Part model, mm, in its own coordinate system. A direction names the side the tool comes from. Give positions to 0.01 mm unless a question says otherwise; leave off trailing zeros. Order: outer loops, then holes, each group sorted by start corner. A loop starts at its lowest first (then second) coordinate and runs counter-clockwise, first axis right, second up.
1. Drop flat-ended pins along their axis: pin 1 Ø4.5 at (x, z) = (4.5, -9) entering from +Y; pin 2 Ø1.5 at (x, z) = (5, 3) entering from -Y; pin 3 Ø4 at (x, y) = (6.5, 3) entering from +Z. Give the stop position or say it passes through.
2. Which spindle directions (+Z, -Z, +X, -X, +Y, -Y) get a long thin tool onto all of the face, cutting with end or side? Do faces 5 (the flat face through (4, 2, -8)), 6 (the cylindrical face through (6.54, -3.81, -10.74)), 7 (the cylindrical face through (3.642, 3.807, -12.414)). Say none if no direction does.
3. Slice it at C-C on x = 5. List the corners of the cut face in (y, z), and give its area (3 significant figures).
4. Slice it at B-B on x = 4. List the corners of the cut face in (y, z), and give its area (3 significant figures).
5. Slice it at D-D on y = 0. List the corners of the cut face in (x, z), and give its area (3 significant figures).
6. Probe line 1 (Z direction, x = 4, y = 2.75); line 2 (Z direction, x = 4, y = 3.9); line 3 (Y direction, x = 3.5, z = -12.5). List the from-to ranges inside material, lowest first.
7. Mould opens along X. For faces 1 (the flat face through (1, 4.3, -11)), 2 (the flat face through (0, -4, -5)), 3 (the cylindrical face through (5.386, -2.659, -10.262)), 4 (the flat face through (5.2, 3.3, -8.5)) say: +X half, -X half, draft (parallel to the pull), parting line (faces both ways), or undercut.
8. Slice it at A-A on z = 0. List the corners of the cut face in (x, y), and give its area (3 significant figures).
Autodesk Inventor part; units mm, degrees
ref_plane "YZ Plane" through (0, 0, 0) normal (1, 0, 0) x (0, 1, 0)
ref_plane "XZ Plane" through (0, 0, 0) normal (0, 1, 0) x (-1, 0, 0)
ref_plane "XY Plane" through (0, 0, 0) normal (0, 0, 1) x (1, 0, 0)
sketch "Sketch2" plane through (0, 0, 0) normal (1, 0, 0) x (0, 1, 0)
  arc A0 (2, -4.8) -> (-2, -4.8) centre (0, 0) ccw
  arc A1 (2, -7.4357) -> (-2, -7.4357) centre (0, 0) ccw
  line L0 (0, 0) -> (2, -4.8)
  line L1 (2, -4.8) -> (2, -7.4357)
  line L2 (2, -7.4357) -> (2, -13.4357)
  line L3 (2, -13.4357) -> (4.3, -13.4357)
  line L4 (4.3, -13.4357) -> (4.3, -6.3875)
  line L5 (0, 0) -> (0, -16.8496) construction
  line L6 (0, 0) -> (-2, -4.8)
  line L7 (-2, -4.8) -> (-2, -7.4357)
  line L8 (-2, -7.4357) -> (-2, -13.4357)
  line L9 (-2, -13.4357) -> (-4.3, -13.4357)
  line L10 (-4.3, -13.4357) -> (-4.3, -6.3875)
  line L11 (-4.3, -6.3875) -> (-2, -6.3875)
  arc A2 (0, -5.2) -> (2, -4.8) centre (0, 0) ccw
  arc A3 (0, -7.7) -> (2, -7.4357) centre (0, 0) ccw
  arc A4 (-2, -7.4357) -> (0, -7.7) centre (0, 0) ccw
  arc A5 (-2, -4.8) -> (0, -5.2) centre (0, 0) ccw
  dimension "d6" = 10.4
  dimension "d7" = 2.5
  dimension "d9" = 2
  dimension "d10" = 6
  dimension "d11" = 2.3
  dimension "d12" = 90
extrude "Extrusion1" add sketch "Sketch2" along normal blind 8 contours A0 L7 L11 A1 L1 | A1 L4 L3 L2 | L7 A1 L11 | L8 L9 L10 A1
sketch "Sketch3" plane through (0, 4.3, -6.3875) normal (0, 1, 0) x (1, 0, 0)
  line L0 (0, 7.0482) -> (0, 0)
  line L1 (0, 0) -> (8, 0)
  line L2 (8, 7.0482) -> (8, 0)
  line L3 (0, 7.0482) -> (8, 7.0482)
  circle A0 centre (4, 3.3) radius 1.5
  point P0 (0, -6.3875)
  dimension "d15" = 3
  dimension "d21" = 3.3
extrude "Extrusion2" cut sketch "Sketch3" against normal up to next contours A0
sketch "Sketch4" plane through (0, 4.3, -6.3875) normal (0, 1, 0) x (1, 0, 0)
  line L0 (0, 7.0482) -> (0, -1.5875)
  line L1 (0, -1.5875) -> (8, -1.5875)
  line L2 (8, 7.0482) -> (8, -1.5875)
  line L3 (0, 7.0482) -> (8, 7.0482)
  circle A0 centre (4, 3.3) radius 1.5
  line L4 (0, 7.0482) -> (0, 0)
  line L5 (0, 0) -> (8, 0)
  line L6 (8, 7.0482) -> (8, 0)
  line L7 (0, 7.0482) -> (8, 7.0482)
  circle A1 centre (4, 3.3) radius 2.75
  point P0 (0, -6.3875)
  dimension "d18" = 5.5
extrude "Extrusion3" cut sketch "Sketch4" against normal blind 1 contours A1
mirror "Mirror1" about plane through (0, 0, 0) normal (0, 1, 0) of "Extrusion3", "Extrusion2"
properties part number "10mm rod Top Clamp"
Data:
1. pin 1: stops at y = 4.3
1. pin 2: stops at y = -7.36
1. pin 3: stops at z = 7.63
2. face 5: -Z, +X, -X
2. face 6: -Y
2. face 7: +Y
3. outline: (-4.3, -13.44) - (-2, -13.44) - (-2, -10.81) - (-3.3, -10.81) - (-3.3, -12.25) - (-4.3, -12.25) - close; (-4.3, -7.13) - (-3.3, -7.13) - (-3.3, -8.57) - (-2, -8.57) - (-2, -4.8) arc R5.2 cw (long way) to (2, -4.8) - (2, -8.57) - (3.3, -8.57) - (3.3, -7.13) - (4.3, -7.13) - (4.3, -6.39) arc R7.7 ccw (long way) to (-4.3, -6.39) - close; (2, -13.44) - (4.3, -13.44) - (4.3, -12.25) - (3.3, -12.25) - (3.3, -10.81) - (2, -10.81) - close
3. area: 105 mm2
4. outline: (-4.3, -13.44) - (-2, -13.44) - (-2, -11.19) - (-3.3, -11.19) - (-3.3, -12.44) - (-4.3, -12.44) - close; (-4.3, -6.94) - (-3.3, -6.94) - (-3.3, -8.19) - (-2, -8.19) - (-2, -4.8) arc R5.2 cw (long way) to (2, -4.8) - (2, -8.19) - (3.3, -8.19) - (3.3, -6.94) - (4.3, -6.94) - (4.3, -6.39) arc R7.7 ccw (long way) to (-4.3, -6.39) - close; (2, -13.44) - (4.3, -13.44) - (4.3, -12.44) - (3.3, -12.44) - (3.3, -11.19) - (2, -11.19) - close
4. area: 102 mm2
5. outline: (0, 5.2) - (8, 5.2) - (8, 7.7) - (0, 7.7) - close
5. area: 20.0 mm2
6. line 1: z = -13.44 to -11.19, -8.19 to -4.41, 4.41 to 7.19
6. line 2: z = -13.44 to -12.44, -6.94 to -3.44, 3.44 to 6.64
6. line 3: y = -4.3 to -2, 2 to 4.3
7. face 1: draft
7. face 2: -X half
7. face 3: undercut
7. face 4: undercut
8. outline: (0, -7.7) - (8, -7.7) - (8, -5.2) - (0, -5.2) - close; (0, 5.2) - (8, 5.2) - (8, 7.7) - (0, 7.7) - close
8. area: 40.0 mm2
